```python
from build123d import *

# Parameters (mm, degrees)
SKETCH1_R           = 150
BOSS_EXTRUDE2_DEPTH = 20
CUT_EXTRUDE1_REACH  = 215.073
SKETCH2_R           = 125
SKETCH3_R           = 137.171463505
BOSS_EXTRUDE3_DEPTH = 59.588855351
BOSS_EXTRUDE4_START = 20
SKETCH4_R           = 150
BOSS_EXTRUDE4_DEPTH = 20
SKETCH6_R           = 125
CUT_EXTRUDE2_DEPTH  = 227.570929062
CUT_EXTRUDE5_REACH  = 236.346
SKETCH7_R           = 1.5


with BuildPart() as part:
    # Sketch1 → Boss-Extrude2 (new body)
    with BuildSketch(Plane.XY):
        Circle(SKETCH1_R)
    extrude(amount=-BOSS_EXTRUDE2_DEPTH)

    # Sketch2 → Cut-Extrude1 (cut, up to next)
    with BuildSketch(Plane(origin=(0, 0, -20), x_dir=(-1, 0, 0), z_dir=(0, 0, -1)), mode=Mode.PRIVATE) as cut_extrude1_sk1:
        Circle(SKETCH2_R)
    cut_extrude1_tool1 = extrude(cut_extrude1_sk1.sketch, amount=-CUT_EXTRUDE1_REACH, mode=Mode.PRIVATE) & part.part
    add(cut_extrude1_tool1.solids().sort_by_distance((0, 0, -20))[0], mode=Mode.SUBTRACT)

    # Sketch3 → Boss-Extrude3 (add)
    with BuildSketch(Plane.XY):
        with Locations(Location((0, 0, 0), (0, 0, 180))):
            Circle(SKETCH3_R)
    extrude(amount=BOSS_EXTRUDE3_DEPTH)

    # Sketch4 → Boss-Extrude4 (add)
    with BuildSketch(Plane.XY.offset(59.588855351).offset(BOSS_EXTRUDE4_START)):
        Circle(SKETCH4_R)
    extrude(amount=-BOSS_EXTRUDE4_DEPTH)

    # Sketch6 → Cut-Extrude2 (cut, through all)
    with BuildSketch(Plane(origin=(0, 0, 0), x_dir=(-1, 0, 0), z_dir=(0, 0, -1))):
        Circle(SKETCH6_R)
    extrude(amount=-CUT_EXTRUDE2_DEPTH, mode=Mode.SUBTRACT)

    # Sketch7 → Cut-Extrude5 (cut, up to next)
    with BuildSketch(Plane.XY.offset(79.588855351), mode=Mode.PRIVATE) as cut_extrude5_sk1:
        with Locations((-145.990171569, 0.381304843)):
            Circle(SKETCH7_R)
    cut_extrude5_tool1 = extrude(cut_extrude5_sk1.sketch, amount=-CUT_EXTRUDE5_REACH, mode=Mode.PRIVATE) & part.part
    add(cut_extrude5_tool1.solids().sort_by_distance((-145.990172, 0.381305, 79.588855))[0], mode=Mode.SUBTRACT)


solid = part.part
```
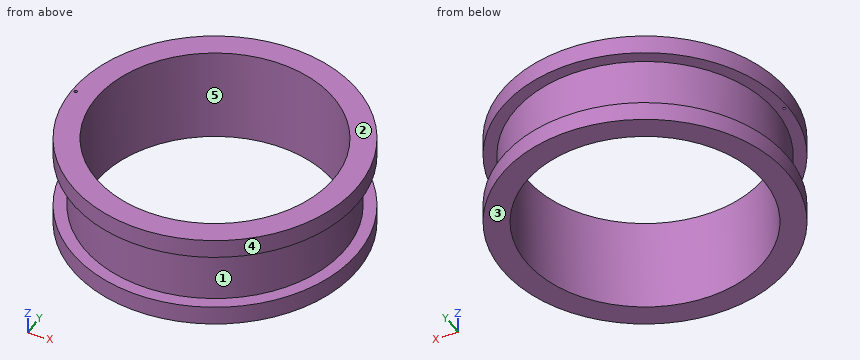
The listing builds one solid part. Answer for the finished solid, in the listing's coordinates (mm). Face numbers are marked on the shaded views. A direction names the side the tool comes from. Give positions to 0.01 mm unless a question says otherwise; leave off trailing zeros. Order: outer loops, then holes, each group sorted by start corner. A loop starts at its lowest first (then second) coordinate and runs counter-clockwise, first axis right, second up. Notation, with made-up numbers: (-39.75, 48.5) -> (12.25, 48.5) arc R17 ccw to (12.25, 52.5) -> close; hole circle Ø10 at (52.25, 49.25). An arc over 180 degrees is marked (long way). Answer as a JSON object with one key per item and string values. Group by question number.
Item 1: The part is cut by section A-A on x = 0. Write down the section's boundary in (y, z), and give its area (3 significant figures).
Item 2: The part is cut by section D-D on z = 36.5. Write down the section's boundary in (x, y), and give its area (3 significant figures).
Item 3: Flat-ended cylindrical pins translate along their axes: pin 1 (4 mm diameter, centred on x = -65.5, z = -3.5, fed in from -Y); pin 2 (2.5 mm diameter, centred on x = -145.99, y = 0.38, fed in from +Z); pin 3 (6 mm diameter, centred on y = -66.5, z = 36.5, fed in from -X); pin 4 (10 mm diameter, centred on x = 11.5, y = -117.5, fed in from +Z). Find the tip coordinate at first contact, or state that the pin passes through.
Item 4: A tool of negligible diameter and unlimited length cuts with its end or side. For the marked faces 1 and 2, from which of +Z, -Z, +X, -X, +Y, -Y can it reach the whole face along a straight path? Write none if from no direction.
Item 5: Determine the mould class of the marked faces 3, 4 and 5 for opening direction Y: pulls with the +Y half, pulls with the -Y half, needs draft (parallel to the pull), parting line crosses it, or undercut.
Item 6: Consider L1, parallel to Z at x = 136, y = 42; L2, parallel to Y at x = 2.5, z = 61 (3 decimals); L3, parallel to Y at x = 0, z = 54.5. Determine where each line is inside the solid, lowest interval first. Write a range as from..to.
Item 7: The part is cut by section C-C on z = -11.5. Write down the section's boundary in (x, y), and give its area (3 significant figures).
Item 8: The part is cut by section B-B on y = -43. Write down the section's boundary in (x, z).
Result set:
{
 "1": {"outline": "(-150, -20) -> (-125, -20) -> (-125, 79.59) -> (-150, 79.59) -> (-150, 59.59) -> (-137.17, 59.59) -> (-137.17, 0) -> (-150, 0) -> close; (125, -20) -> (150, -20) -> (150, 0) -> (137.17, 0) -> (137.17, 59.59) -> (150, 59.59) -> (150, 79.59) -> (125, 79.59) -> close", "area": "3,450 mm²"},
 "2": {"outline": "circle Ø274.34 at (0, 0); hole circle Ø250 at (0, 0)", "area": "10,000 mm²"},
 "3": {"pin 1": "y = -135.9", "pin 2": "z = 0", "pin 3": "x = -121.59", "pin 4": "through"},
 "4": {"face 1": "none", "face 2": "+Z, +X, -X, +Y, -Y"},
 "5": {"face 3": "needs draft", "face 4": "parting line crosses it", "face 5": "undercut"},
 "6": {"L1": "-20..0, 59.59..79.59", "L2": "-149.979..-124.975, 124.975..149.979", "L3": "-137.17..-125, 125..137.17"},
 "7": {"outline": "circle Ø300 at (0, 0); hole circle Ø250 at (0, 0)", "area": "21,600 mm²"},
 "8": {"outline": "(-143.7, -20) -> (-117.37, -20) -> (-117.37, 79.59) -> (-143.7, 79.59) -> (-143.7, 59.59) -> (-130.26, 59.59) -> (-130.26, 0) -> (-143.7, 0) -> close; (117.37, -20) -> (143.7, -20) -> (143.7, 0) -> (130.26, 0) -> (130.26, 59.59) -> (143.7, 59.59) -> (143.7, 79.59) -> (117.37, 79.59) -> close"}
}
